Source: CAD feature listing. Evaluate the final solid. Frame: model axes, mm. A direction names the side the tool comes from. Round coordinates to 2 decimals unless told otherwise and drop trailing zeros. Write item = value, one per line. Start each with the question number.
(1) Contact query for flat-ended pins moving along their axis: pin 1 Ø2 at (x, y) = (-5.5, -1) entering from +Z; pin 2 Ø6.5 at (x, z) = (24.75, -24.75) entering from -Y; pin 3 Ø2 at (x, y) = (-20.5, 1) entering from -Z. Output: stop coordinate, or through.
(2) Reachability of faces 1 (the face through (37.727, 2.542, -0.358)), 2 (the face through (-32.8, -0.5, -2.2)), 3 (the face through (18.2, 3.5, -14.4)) from +Z, -Z, +X, -X, +Y, -Y: full face, straight path, thin tool, end or side. Return the list, or none.
(3) Cut plane A-A on x = 0. Give the number of separate pieces and of enclosed holes in the cut face, then the cut area to 3 significant figures.
(4) Ray query, line 1 (Z direction, x = -23.5, y = 0.25); line 2 (X direction, y = 4.25, z = -9.5); line 3 (Y direction, x = 23, z = -22.5). Return the intervals inside material, ascending.
(5) Draft query along Z for faces 4 (the face through (-0.358, 2.542, -37.727)), 5 (the face through (-20, 5.5, 21)), 6 (the face through (36.107, 1.063, -27.686)). Return one class per face: released by +Z, released by -Z, zero draft, split by the parting line, or undercut.
Autodesk Inventor part; units mm, degrees
ref_plane "YZ Plane" through (0, 0, 0) normal (1, 0, 0) x (0, 1, 0)
ref_plane "XZ Plane" through (0, 0, 0) normal (0, 1, 0) x (-1, 0, 0)
ref_plane "XY Plane" through (0, 0, 0) normal (0, 0, 1) x (1, 0, 0)
sketch "Sketch1" plane through (0, 0, 0) normal (0, 1, 0) x (-1, 0, 0)
  circle A0 centre (0, 0) radius 45.5
  dimension "d0" = 91
extrude "Extrusion1" add sketch "Sketch1" along normal mid plane 11
fillet "Fillet1" radius 2 1 edges at (45.5, -5.5, 0)
hole "Hole1" at (0, 5.5, 0) direction (0, -1, 0) diameter 46 end through all
hole "Hole2" at (0, 5.5, 0) direction (0, -1, 0) diameter 55 depth 2
fillet "Fillet2" radius 1 1 edges at (0, 5.5, -27.5)
sketch "Sketch2" plane through (0, -5.5, 0) normal (0, 1, 0) x (1, 0, 0)
  line L0 (-35, 0) -> (0, 0) construction
  dimension "d23" = 35
hole "Hole3" at (-35, -5.5, 0) direction (0, 1, 0) diameter 5.5 end through all counterbore diameter 10 counterbore depth 5
pattern_circular "Circular Pattern2" count 8 over 360 about axis through (0, -123.6627, 0) along (0, 1, 0) of "Hole3"
properties part number "301-06" material "Stainless Steel"
Evaluation:
q1.pin_1 = 45.28
q1.pin_2 = -0.5
q1.pin_3 = -41.11
q2.face_1 = +Y, -Y
q2.face_2 = -Y
q2.face_3 = +Y
q3.separate_pieces = 4
q3.enclosed_holes = 0
q3.area = 309 mm^2
q4.line_1 = -38.96 to -27.2, -22.3 to 22.3, 27.2 to 38.96
q4.line_2 = -44.5 to -25.81, 25.81 to 44.5
q4.line_3 = -0.5 to 5.5
q5.face_4 = undercut
q5.face_5 = zero draft
q5.face_6 = split by the parting line
